```python
from build123d import *

# Parameters (mm, degrees)
F0_R          = 19
F1_DEPTH      = 16
F2_R          = 1.74
F3_DEPTH      = 19.001
F3_DEPTH_BACK = 19.001
F4_R          = 1.9835
F5_DEPTH      = 16.0010001


with BuildPart() as f1:
    # F0 (on Top) → F1 (new body)
    with BuildSketch(Plane.XY):
        Circle(F0_R)
    extrude(amount=F1_DEPTH)

    # F2 (on Right) → F3 (cut, two sides)
    with BuildSketch(Plane.YZ) as f3_sk:
        with Locations((0, 14.8)):
            Circle(F2_R)
    extrude(amount=-F3_DEPTH, mode=Mode.SUBTRACT)
    extrude(f3_sk.sketch, amount=F3_DEPTH_BACK, mode=Mode.SUBTRACT)

    # F4 (on Top) → F5 (cut, through all)
    with BuildSketch(Plane.XY):
        with Locations((11.2, -6.25)):
            Circle(F4_R)
        with Locations((11.2, 6.25)):
            Circle(F4_R)
    extrude(amount=F5_DEPTH, mode=Mode.SUBTRACT)


solid = f1.part
```
The model under review builds one solid part; all positions refer to its coordinate system, in mm. Round coordinates to 2 decimals unless told otherwise and drop trailing zeros. Loops run counter-clockwise (first coordinate to the right, second up) from the corner with the lowest first, then second, coordinate; pieces in that order, holes last. Notation, with made-up numbers: M 44,27 L 100,27 A7 ccw 100,33 Z; hole C 59.25,39 d9. An arc over 180 degrees is marked long. Write item = value, one per line.
Item 1: Take a section at C-C on x = 11.2. Write out the cut boundary in (y, z), then the cut area to 3 significant figures.
Return value:
outline = M -15.35,0 L -8.23,0 L -8.23,16 L -15.35,16 Z; M -4.27,0 L 4.27,0 L 4.27,16 L 1.26,16 A1.74 cw long -1.26,16 L -4.27,16 Z; M 8.23,0 L 15.35,0 L 15.35,16 L 8.23,16 Z
area = 356 mm2
Item 2: Take a section at B-B on y = -5. Write out the cut boundary in (x, z), then the cut area to 3 significant figures.
Return value:
outline = M -18.33,0 L 9.66,0 L 9.66,16 L -18.33,16 Z; M 12.74,0 L 18.33,0 L 18.33,16 L 12.74,16 Z
area = 537 mm2
Item 3: Insertion check: P1, Ø3, axis at x = 2, z = 2, coming from the +Y side; P2, Ø3, axis at x = 5.5, z = 3, coming from the -Y side; P3, Ø1, axis at x = 2.5, z = 9, coming from the -Y side; P4, Ø3, axis at y = 0, z = 14.8, coming from the -X side. Each pin has a flat end and moves straight along its axis. Give the tip position at first contact, or say it passes through.
Return value:
P1 = 18.99
P2 = -18.57
P3 = -18.89
P4 = through
Item 4: For line 1 (Y direction, x = 11.2, z = 8.25); line 2 (Y direction, x = 11, z = 14); line 3 (Y direction, x = 0.5, z = 15.25), list the stretches that pass through material, from the lowest coordinate up. Write a range as [from, to].
Return value:
line_1 = [-15.35, -8.23], [-4.27, 4.27], [8.23, 15.35]
line_2 = [-15.49, -8.22], [-4.28, -1.55], [1.55, 4.28], [8.22, 15.49]
line_3 = [-18.99, -1.68], [1.68, 18.99]
Item 5: The part is to be moulded in two halves that separate along Y. For faces 1 (the cylindrical face through (13.09, -5.65, 7.89)), 2 (the flat face through (0, 8, 16)), 3 (the cylindrical face through (17.55, -7.28, 7.89)), say which applies: released by +Y, released by -Y, zero draft, split by the parting line, or undercut.
Return value:
face_1 = undercut
face_2 = zero draft
face_3 = split by the parting line
Item 6: Take a section at D-D on x = -4.5. Write out the cut boundary in (y, z), then the cut area to 3 significant figures.
Return value:
outline = M -18.46,0 L 18.46,0 L 18.46,16 L 1.26,16 A1.74 cw long -1.26,16 L -18.46,16 Z
area = 582 mm2
Item 7: Take a section at A-A on z = 13.75. Write out the cut boundary in (x, y).
Return value:
outline = M -18.95,-1.39 A19 ccw 18.95,-1.39 Z; M -18.95,1.39 L 18.95,1.39 A19 ccw Z; hole C 11.2,-6.25 d3.97; hole C 11.2,6.25 d3.97
